Here's the drawing with two shaded views (mm, measured from the low corner). I have some questions. A direction names the side the tool comes from. Give positions to 0.01 mm unless a question says otherwise; leave off trailing zeros. Order: outer loops, then holes, each group sorted by start corner. A loop starts at its lowest first (then second) coordinate and runs counter-clockwise, first axis right, second up. Notation, with made-up numbers: M -15,-32 L 5,-32 A29 cw 5,4 Z; hole C -18,-0.5 d1. An arc over 180 degrees is marked long. Use a Markdown table: item, result. Add a question column.
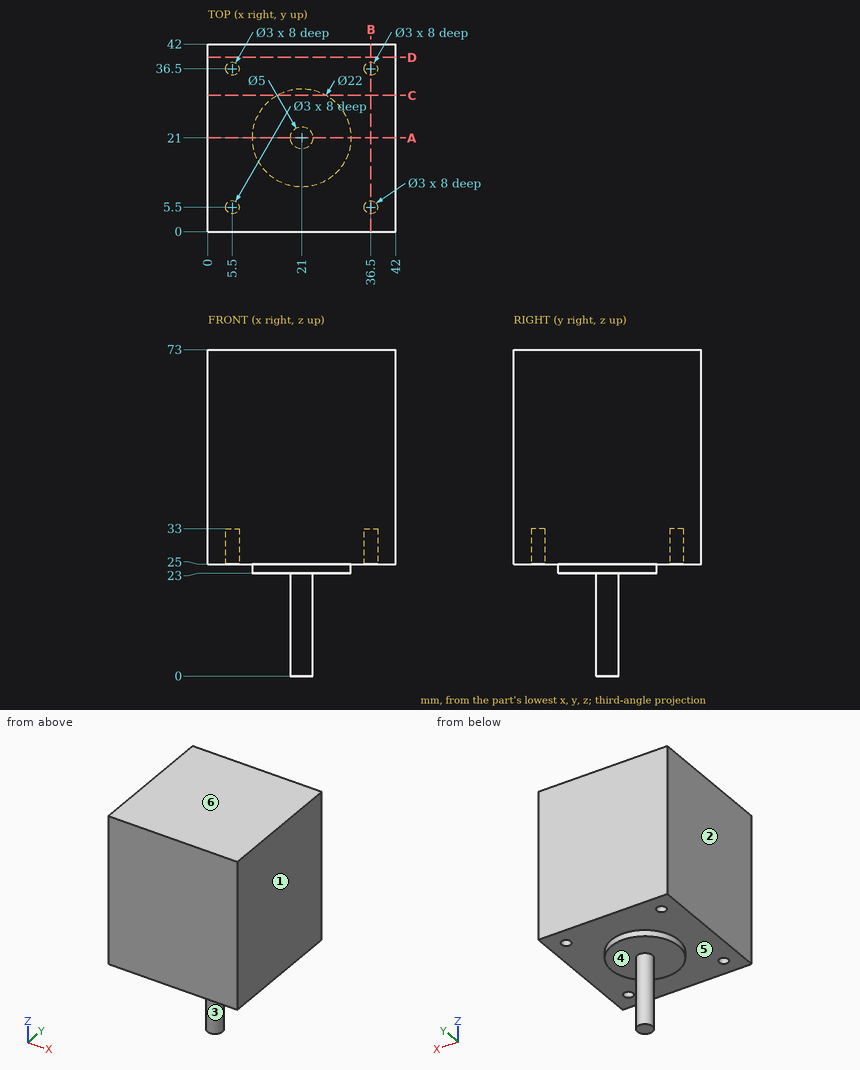
1. On a 3-axis mill with a long thin cutter (end or side, diameter ignored), from which of +Z, -Z, +X, -X, +Y, -Y can I reach the whole of each face in a straight line? I mean the marked faces 5 and 6. Say none if no direction works.
2. If we section it at A-A, the plane y = 21: List the corners of the cut face in (x, z) for me, then the cut area to 4 significant figures.
3. If we section it at D-D, the plane y = 39: List the corners of the cut face in (x, z) for me, then the cut area to 3 significant figures.
4. Will these pins go through, and if not, where does the flat tip stop? pin 1 (2.5 mm diameter, centred on x = 36, y = 36, fed in from -Z); pin 2 (6.5 mm diameter, centred on x = 18.5, y = 24, fed in from -Z); pin 3 (2.5 mm diameter, centred on x = 36.5, y = 36.5, fed in from -Z).
5. We'd pull the mould along X, two halves only. Please class the marked faces 1, 2, 3 and 4: +X half, -X half, draft (parallel to the pull), parting line (faces both ways), or undercut.
6. If we section it at C-C, the plane y = 30.5: List the corners of the cut face in (x, z) for me, then the cut area to 3 significant figures.
7. I need wall thicknesses on L1, parallel to X at y = 36, z = 30; L2, parallel to Z at x = 18, y = 21. Which ranges of each line are inside material? Lowest first, please. Write a range as [from, to].
8. If we section it at B-B, the plane x = 36.5: List the corners of the cut face in (y, z) for me, then the cut area to 3 significant figures.
Geometry results:
| question | item | result |
|---|---|---|
| 1 | face 5 | -Z |
| 1 | face 6 | +Z, +X, -X, +Y, -Y |
| 2 | outline | M 0,25 L 10,25 L 10,23 L 18.5,23 L 18.5,0 L 23.5,0 L 23.5,23 L 32,23 L 32,25 L 42,25 L 42,73 L 0,73 Z |
| 2 | area | 2,175 mm^2 |
| 3 | outline | M 0,25 L 42,25 L 42,73 L 0,73 Z |
| 3 | area | 2,020 mm^2 |
| 4 | pin 1 | stops at z = 25 |
| 4 | pin 2 | stops at z = 0 |
| 4 | pin 3 | stops at z = 33 |
| 5 | face 1 | +X half |
| 5 | face 2 | -X half |
| 5 | face 3 | parting line |
| 5 | face 4 | draft |
| 6 | outline | M 0,25 L 15.45,25 L 15.45,23 L 26.55,23 L 26.55,25 L 42,25 L 42,73 L 0,73 Z |
| 6 | area | 2,040 mm^2 |
| 7 | L1 | x = [0, 4.09], [6.91, 35.09], [37.91, 42] |
| 7 | L2 | z = [23, 73] |
| 8 | outline | M 0,25 L 4,25 L 4,33 L 7,33 L 7,25 L 35,25 L 35,33 L 38,33 L 38,25 L 42,25 L 42,73 L 0,73 Z |
| 8 | area | 1,970 mm^2 |
